```python
from build123d import *

# Parameters (mm, degrees)
SKETCH_2_W                = 40
SKETCH_2_H                = 22.5
EXTRUDE_2_DEPTH           = 25
SHELL_3_T                 = -1
CUT_EXTRUDE_2_DEPTH       = 56.37502058
CUT_EXTRUDE_2_DEPTH_BACK  = 1
CUT_EXTRUDE_10_DEPTH      = 56.37502058
CUT_EXTRUDE_10_DEPTH_BACK = 1
SKETCH_6_W                = 40
SKETCH_6_H                = 22.5
EXTRUDE_3_DEPTH           = 10


with BuildPart() as part:
    # 草图2 → 凸台-拉伸2 (new body)
    with BuildSketch(Plane(origin=(0, 0, 0), x_dir=(1, 0, 0), z_dir=(0, 1, 0))):
        with Locations((-23.990259198, 8.7812953)):
            Rectangle(SKETCH_2_W, SKETCH_2_H)
    extrude(amount=EXTRUDE_2_DEPTH)

    # 抽壳3
    shell_3_openings = [part.faces().sort_by_distance(p)[0] for p in [
        (-23.990259198, 0, -8.7812953),
        (-3.990259198, 12.5, -8.7812953),
        (-43.990259198, 12.5, -8.7812953),
    ]]
    offset(amount=SHELL_3_T, openings=shell_3_openings, kind=Kind.INTERSECTION)

    # 草图4 → 切除-拉伸2 (cut, two sides: drawn at the far end of the back side and taken through both)
    with BuildSketch(Plane.XY.offset(2.4687047).offset(-CUT_EXTRUDE_2_DEPTH_BACK)):
        with BuildLine():
            Line((-24.990259198, 12), (-24.990259198, 0))
            Line((-24.990259198, 0), (-35.990259198, 0))
            Line((-35.990259198, 0), (-35.990259198, 12))
            ThreePointArc((-35.990259198, 12), (-30.490259198, 17.5), (-24.990259198, 12))
        make_face()
        with BuildLine():
            Line((-21.490259198, 12), (-21.490259198, 0))
            Line((-21.490259198, 0), (-17.490259198, 0))
            Line((-17.490259198, 0), (-17.490259198, 12))
            ThreePointArc((-17.490259198, 12), (-19.490259198, 14), (-21.490259198, 12))
        make_face()
    extrude(amount=CUT_EXTRUDE_2_DEPTH + CUT_EXTRUDE_2_DEPTH_BACK, mode=Mode.SUBTRACT)

    # 草图5 → 切除-拉伸10 (cut, two sides: drawn at the far end of the back side and taken through both)
    with BuildSketch(Plane(origin=(0, 0, -20.0312953), x_dir=(-1, 0, 0), z_dir=(0, 0, -1)).offset(-CUT_EXTRUDE_10_DEPTH_BACK)):
        with BuildLine():
            Line((35.990259198, 12), (35.990259198, 0))
            Line((35.990259198, 0), (24.990259198, 0))
            Line((24.990259198, 0), (24.990259198, 12))
            ThreePointArc((24.990259198, 12), (30.490259198, 17.5), (35.990259198, 12))
        make_face()
        with BuildLine():
            Line((17.490259198, 12), (17.490259198, 0))
            Line((17.490259198, 0), (21.490259198, 0))
            Line((21.490259198, 0), (21.490259198, 12))
            ThreePointArc((21.490259198, 12), (19.490259198, 14), (17.490259198, 12))
        make_face()
    extrude(amount=CUT_EXTRUDE_10_DEPTH + CUT_EXTRUDE_10_DEPTH_BACK, mode=Mode.SUBTRACT)

    # 草图6 → 凸台-拉伸3 (add)
    with BuildSketch(Plane(origin=(0, 25, 0), x_dir=(1, 0, 0), z_dir=(0, 1, 0))):
        with Locations((-23.990259198, 8.7812953)):
            Rectangle(SKETCH_6_W, SKETCH_6_H)
    extrude(amount=EXTRUDE_3_DEPTH)


solid = part.part
```
Geometry check sheet. Reference: the model listing, model coordinates, mm. A direction names the side the tool comes from. Coordinates: 2 decimals unless noted, no trailing zeros. Order: outer loops, then holes, each group sorted by start corner. A loop starts at its lowest first (then second) coordinate and runs counter-clockwise, first axis right, second up. Notation, with made-up numbers: (-30.75, 25) - (25.25, 25) arc R25 cw to (25.25, 55) - close; hole circle Ø5 at (44, 82). An arc over 180 degrees is marked (long way). Use one line per item in the form item = value.
1. Access from +Z, -Z, +X, -X, +Y, -Y to the whole of each face (thin tool, end or side, straight path). Record for faces 1 (the face through (-24, 12, -19.031)), 2 (the face through (-24, 17, 2.469)), 3 (the face through (-24.99, 6, 2)).
Here are the results:
face_1 = +X, -X, -Y
face_2 = +Z, +X, -X, +Y, -Y
face_3 = +Z, -Z, -Y
2. Section check D-D (x = -35). Record the boundary of the cut face in (y, z), then the cut area to 3 significant figures.
Here are the results:
outline = (15.15, -20.03) - (35, -20.03) - (35, 2.47) - (15.15, 2.47) - (15.15, 1.47) - (24, 1.47) - (24, -19.03) - (15.15, -19.03) - close
area = 265 mm²
3. Scan lines: line 1 (Z direction, x = -11, y = 12.5); line 2 (Y direction, x = -41.5, z = -17.5). Record each from-to range of solid material in increasing order.
Here are the results:
line_1 = -20.03 to -19.03, 1.47 to 2.47
line_2 = 24 to 35
4. Section check A-A (x = -13.5). Record the boundary of the cut face in (y, z), then the cut area to 4 significant figures.
Here are the results:
outline = (0, -20.03) - (35, -20.03) - (35, 2.47) - (0, 2.47) - (0, 1.47) - (24, 1.47) - (24, -19.03) - (0, -19.03) - close
area = 295.5 mm²
5. Section check C-C (z = 0.25). Record the boundary of the cut face in (x, y).
Here are the results:
outline = (-43.99, 24) - (-3.99, 24) - (-3.99, 35) - (-43.99, 35) - close
6. Draft check along X on faces 4 (the face through (-40, 0, -19.5)), 5 (the face through (-3.99, 28, -10)), 6 (the face through (-17.49, 6, 2)). Enter one of: pulls with the +X half, pulls with the -X half, needs draft (parallel to the pull), parting line crosses it, or undercut.
Here are the results:
face_4 = needs draft
face_5 = pulls with the +X half
face_6 = undercut
7. Section check B-B (y = 16). Record the boundary of the cut face in (x, z), then the cut area to 3 significant figures.
Here are the results:
outline = (-43.99, -20.03) - (-34.27, -20.03) - (-34.27, -19.03) - (-43.99, -19.03) - close; (-43.99, 1.47) - (-34.27, 1.47) - (-34.27, 2.47) - (-43.99, 2.47) - close; (-26.72, -20.03) - (-3.99, -20.03) - (-3.99, -19.03) - (-26.72, -19.03) - close; (-26.72, 1.47) - (-3.99, 1.47) - (-3.99, 2.47) - (-26.72, 2.47) - close
area = 64.9 mm²
8. Gauge pin test, flat end, axial feed: pin 1 (6 mm diameter, centred on x = -25, z = -11, fed in from -Y). Record the tip position at first contact, or that the pin passes through.
Here are the results:
pin_1 = 24
